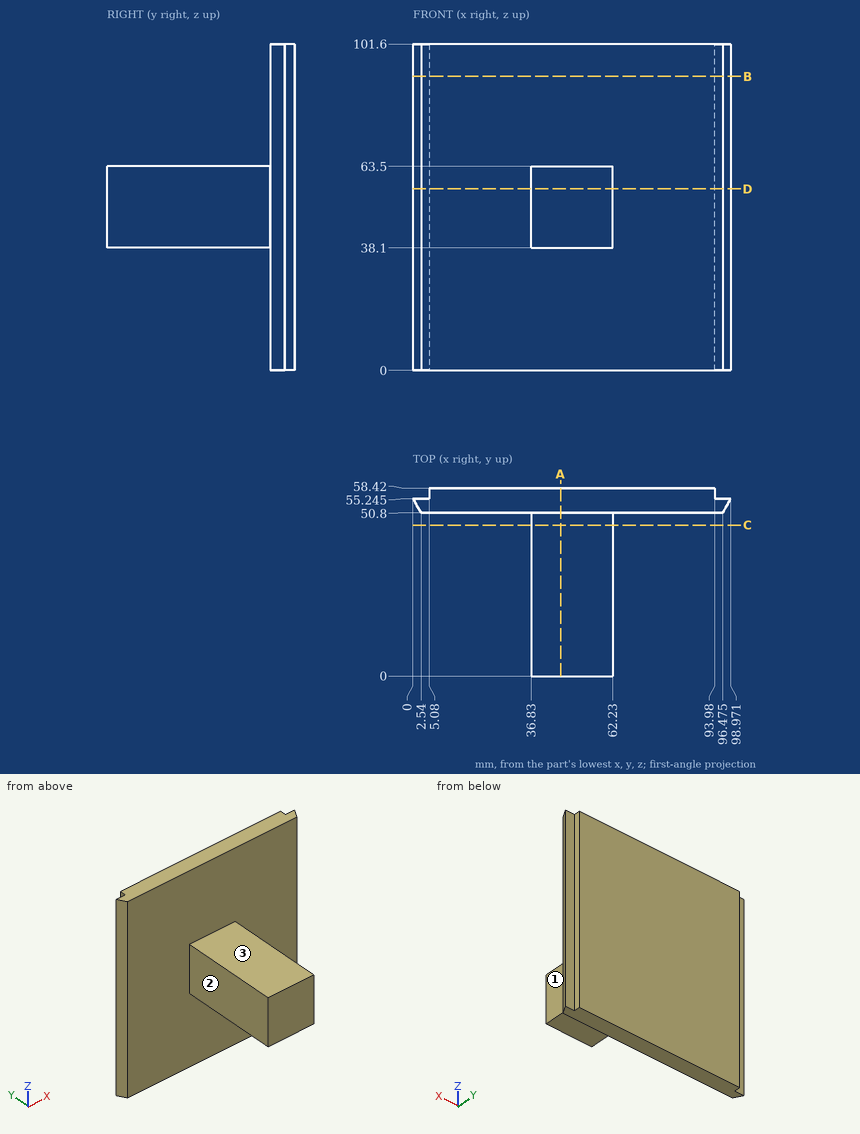
Drawing for the job (mm, zero at the part's lowest x, y, z). A direction names the side the tool comes from. Give positions to 0.01 mm unless a question says otherwise; leave off trailing zeros. Order: outer loops, then holes, each group sorted by start corner. A loop starts at its lowest first (then second) coordinate and runs counter-clockwise, first axis right, second up. Notation, with made-up numbers: M 24,-7.5 L 79,-7.5 A22 cw 79,9.5 Z; hole C 80,85 d5. An arc over 180 degrees is marked long. Use a Markdown table: item, result. Add a question column.
(1) Saw through at D-D, the plane z = 56.5. Give the cut face in (x, y) (1 decimal), and give its area (3 significant figures).
(2) Saw through at A-A, the plane x = 46. Give the cut face in (y, z), and give its area (3 significant figures).
(3) Saw through at B-B, the plane z = 91.5. Give the cut face in (x, y) (1 decimal).
(4) Saw through at C-C, the plane y = 47. Give the cut face in (x, z).
(5) Drop flat-ended pins along their axis: P1, Ø12.5, axis at y = 18.5, z = 49, coming from the -X side; P2, Ø20.5, axis at x = 53, y = 16.5, coming from the +Z side; P3, Ø2.5, axis at y = 56, z = 62, coming from the +X side; P4, Ø3, axis at x = 73, z = 65, coming from the -Y side. Give the stop position or say it passes through.
(6) Probe line 1 along Y through (x, z) = (15, 61.5); line 2 along Z through (x, y) = (40.5, 24); line 3 along Y through (x, z) = (95.5, 49) (1 decimal). List the from-to ranges inside material, lowest first. Write a range as [from, to].
(7) 3-axis set-ups, long thin cutter, end or side, ignore diameter. For the marked faces 1, 2 and 3: which of +Z, -Z, +X, -X, +Y, -Y reach the whole face in a straight line?
Answer key:
| question | item | result |
|---|---|---|
| 1 | outline | M 0,55.2 L 2.5,50.8 L 36.8,50.8 L 36.8,0 L 62.2,0 L 62.2,50.8 L 96.5,50.8 L 99,55.2 L 94,55.2 L 94,58.4 L 5.1,58.4 L 5.1,55.2 Z |
| 1 | area | 2,000 mm^2 |
| 2 | outline | M 0,38.1 L 50.8,38.1 L 50.8,0 L 58.42,0 L 58.42,101.6 L 50.8,101.6 L 50.8,63.5 L 0,63.5 Z |
| 2 | area | 2,060 mm^2 |
| 3 | outline | M 0,55.2 L 2.5,50.8 L 96.5,50.8 L 99,55.2 L 94,55.2 L 94,58.4 L 5.1,58.4 L 5.1,55.2 Z |
| 4 | outline | M 36.83,38.1 L 62.23,38.1 L 62.23,63.5 L 36.83,63.5 Z |
| 5 | P1 | x = 36.83 |
| 5 | P2 | z = 63.5 |
| 5 | P3 | x = 98.97 |
| 5 | P4 | y = 50.8 |
| 6 | line 1 | [50.8, 58.42] |
| 6 | line 2 | [38.1, 63.5] |
| 6 | line 3 | [50.8, 55.2] |
| 7 | face 1 | +Z, -Z, +X, -Y |
| 7 | face 2 | +Z, -Z, -X, -Y |
| 7 | face 3 | +Z, +X, -X, -Y |
